Check sheet for the drawn part. Datum: minimum x, y, z corner. Units: mm. A direction names the side the tool comes from. Give positions to 0.01 mm unless a question says otherwise; leave off trailing zeros. Write each loop counter-clockwise with the first axis right and the second up, starting at its lowest first coordinate (ties: lowest second). Pieces come first, ordered by that corner, then holes. Notation, with made-up numbers: (57.25, 35) - (63.25, 35) arc R27 cw to (63.25, 64) - close; hole circle Ø11 at (-1, -15). An arc over 180 degrees is marked (long way). One line per question, with ' | ' between items. Start each with the question number.
Q1. Gauge pin test, flat ends, axial feed: P1, Ø1, axis at x = 28.5, z = 13, coming from the -Y side (1 decimal); P2, Ø2.5, axis at x = 3.5, y = 15, coming from the -Z side; P3, Ø4.5, axis at x = 38, y = 23.5, coming from the +Z side. Record the tip position at first contact, or that the pin passes through.
Q2. Set-up check for the marked faces 4, 5, 6 and 7: record each of +Z, -Z, +X, -X, +Y, -Y from which the full face is reachable in a straight line by a thin tool's end or side.
Q3. Section check C-C on x = 23. Record the boundary of the cut face in (y, z) (1 decimal), and give its area (3 significant figures).
Q4. Section check A-A on y = 26.5. Record the boundary of the cut face in (x, z), and give its area (3 significant figures).
Q5. Thickness scan on L1, parallel to X at y = 21.5, z = 6.75; L2, parallel to Y at x = 8, z = 7.5; L3, parallel to Y at x = 31, z = 19.75. Record the ranges inside material, lowest first. Write a range as [from, to].
Q6. Release check for a two-part mould opening along X. For the marked faces 1, 2 and 3 record: +X half, -X half, draft (parallel to the pull), parting line (faces both ways), or undercut.
Q7. Section check B-B on z = 3.75. Record the boundary of the cut face in (x, y).
Q8. Section check D-D on x = 35.5. Record the boundary of the cut face in (y, z) (1 decimal).
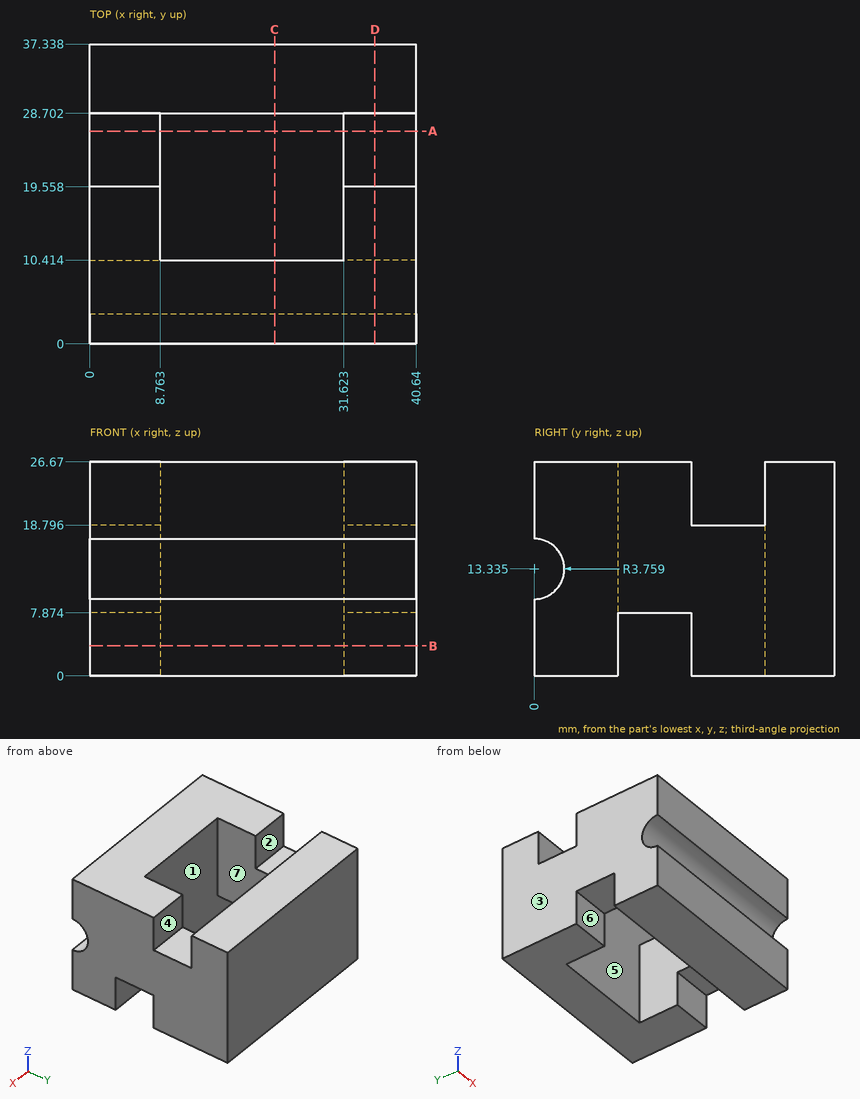
Working result:
1) P1: stops at y = 3.7 | P2: stops at z = 7.87 | P3: stops at z = 18.8
2) face 4: +Z, +X, -X | face 5: +Z | face 6: -Z, +X, -X | face 7: +Z, -Z
3) outline: (0, 0) - (10.4, 0) - (10.4, 26.7) - (0, 26.7) - (0, 17.1) arc R3.8 cw to (0, 9.6) - close; (28.7, 0) - (37.3, 0) - (37.3, 26.7) - (28.7, 26.7) - close | area: 486 mm2
4) outline: (0, 0) - (8.76, 0) - (8.76, 18.8) - (0, 18.8) - close; (31.62, 0) - (40.64, 0) - (40.64, 18.8) - (31.62, 18.8) - close | area: 334 mm2
5) L1: x = [0, 8.76], [31.62, 40.64] | L2: y = [0, 10.41], [19.56, 37.34] | L3: y = [0, 10.41], [28.7, 37.34]
6) face 1: undercut | face 2: draft | face 3: -X half
7) outline: (0, 0) - (40.64, 0) - (40.64, 10.41) - (0, 10.41) - close; (0, 19.56) - (8.76, 19.56) - (8.76, 28.7) - (31.62, 28.7) - (31.62, 19.56) - (40.64, 19.56) - (40.64, 37.34) - (0, 37.34) - close
8) outline: (0, 0) - (10.4, 0) - (10.4, 7.9) - (19.6, 7.9) - (19.6, 0) - (37.3, 0) - (37.3, 26.7) - (28.7, 26.7) - (28.7, 18.8) - (19.6, 18.8) - (19.6, 26.7) - (0, 26.7) - (0, 17.1) arc R3.8 cw to (0, 9.6) - close
